Geometry: see drawing. Coordinates: mm, zero at the bounding-box minimum. Give positions to 0.01 mm unless a question says otherwise; leave off trailing zeros. Write each loop counter-clockwise with the first axis right and the second up, starting at its lowest first coordinate (ties: lowest second). Pieces come first, ordered by that corner, then holes. Notation, with made-up numbers: (-24, 26) - (16, 26) arc R17 ccw to (16, 59) - close; hole circle Ø3 at (-7, -18). An arc over 180 degrees is marked (long way). Use CSV: the item, a comma, the result in double quotes. Start each with the question number.
(1) Section C-C on x = 34.5. Output: boundary loops of the cut face in (y, z) (1 decimal), and give its area (3 significant figures).
(2) Section D-D on y = 18.5. Output: boundary loops of the cut face in (x, z) (1 decimal).
(3) Section A-A on x = 24.5. Output: boundary loops of the cut face in (y, z) (1 decimal).
(4) Line query: probe 1 along Y at (x, z) = (24, 1.6); probe 2 along Y at (x, z) = (13, 1.2) (1 decimal); probe 3 along X at (y, z) = (32, 1.4) (1 decimal). Output: solid intervals per line, ascending. Write a range as [from, to].
(5) First-contact query: pin 1 Ø1.6 at (y, z) = (2, 2) entering from -X; pin 2 Ø10 at (x, y) = (12, 18) entering from -Z; pin 3 Ø1 at (y, z) = (2, 1.5) entering from +X; pin 4 Ø3 at (x, y) = (23.81, 30.73) entering from +Z. Flat tips, straight axial feed; report the tip coordinate or a pass-through.
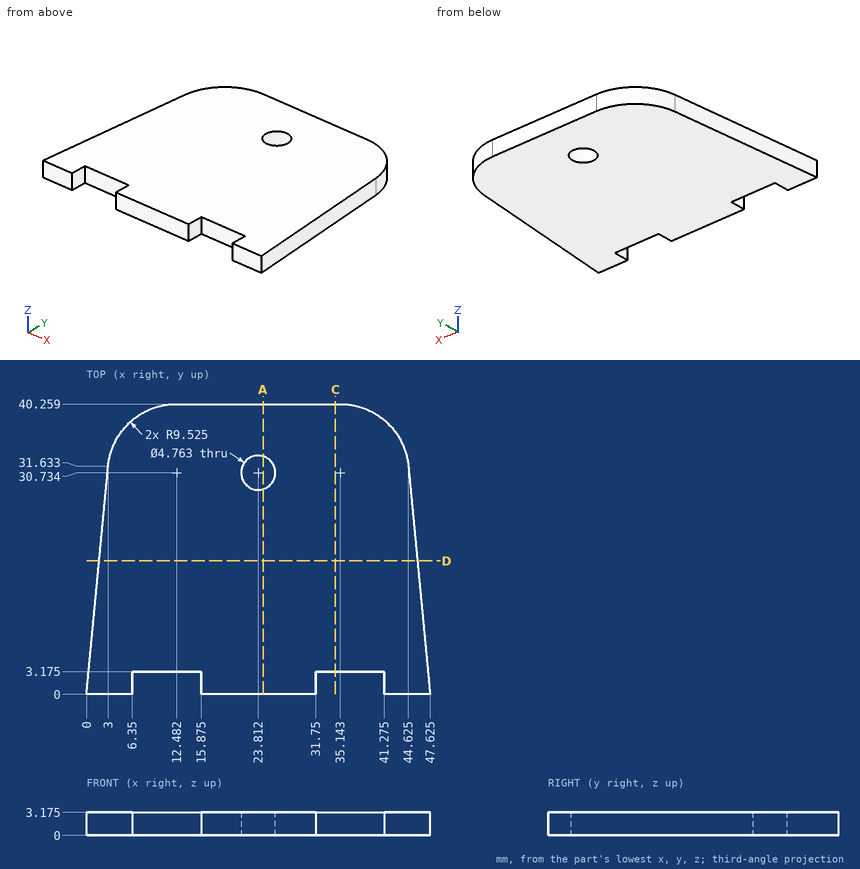
Check values:
1,outline,"(3.2, 0) - (40.3, 0) - (40.3, 3.2) - (3.2, 3.2) - close"
1,area,"118 mm²"
2,outline,"(1.8, 0) - (45.9, 0) - (45.9, 3.2) - (1.8, 3.2) - close"
3,outline,"(0, 0) - (28.5, 0) - (28.5, 3.2) - (0, 3.2) - close; (33, 0) - (40.3, 0) - (40.3, 3.2) - (33, 3.2) - close"
4,probe 1,"y = [0, 28.36], [33.11, 40.26]"
4,probe 2,"y = [3.2, 40.3]"
4,probe 3,"x = [3, 21.8], [25.8, 44.6]"
5,pin 1,"stops at x = 0.11"
5,pin 2,"stops at z = 0"
5,pin 3,"stops at x = 47.48"
5,pin 4,"passes through"
